CAD build for the part. Positions are in the model's coordinates, mm. Face numbers are marked on the shaded views. A direction names the side the tool comes from. Round coordinates to 2 decimals unless told otherwise and drop trailing zeros. Loops run counter-clockwise (first coordinate to the right, second up) from the corner with the lowest first, then second, coordinate; pieces in that order, holes last. Notation, with made-up numbers: (38.25, -19.5) - (81.25, -19.5) arc R8 cw to (81.25, -10.5) - close; hole circle Ø5 at (-24, 64). An arc over 180 degrees is marked (long way). Use one line per item in the form item = value.
from build123d import *

# Parameters (mm, degrees)
F0_W     = 5.15
F0_H     = 7
F1_DEPTH = 6.74
F2_R     = 1.3
F3_DEPTH = 25
F4_R     = 0.8
F5_DEPTH = 6.741


with BuildPart() as f1:
    # F0 (on Front) → F1 (new body)
    with BuildSketch(Plane.XZ):
        with BuildLine():
            Line((7, 2.5), (-7, 2.5))
            ThreePointArc((-7, 2.5), (-8.06066, 2.06066), (-8.5, 1))
            Line((-8.5, 1), (-8.5, -2.5))
            Line((-8.5, -2.5), (-3.35, -2.5))
            Line((-3.35, -2.5), (3.35, -2.5))
            Line((3.35, -2.5), (8.5, -2.5))
            Line((8.5, -2.5), (8.5, 1))
            ThreePointArc((8.5, 1), (8.06066, 2.06066), (7, 2.5))
        make_face()
        with Locations((-5.925, -6)):
            Rectangle(F0_W, F0_H)
        with Locations((5.925, -6)):
            Rectangle(F0_W, F0_H)
    extrude(amount=F1_DEPTH)

    # F2 (on face) → F3 (cut)
    with BuildSketch(Plane.XZ.offset(6.74)):
        with Locations((-2.6, -3.25)):
            Circle(F2_R)
        with Locations((2.6, -3.25)):
            Circle(F2_R)
    extrude(amount=-F3_DEPTH, mode=Mode.SUBTRACT)

    # F4 (on face) → F5 (cut, through all)
    with BuildSketch(Plane.XZ.offset(6.74)):
        with Locations((-5.925, -4.5)):
            Circle(F4_R)
        with Locations((5.925, -4.5)):
            Circle(F4_R)
    extrude(amount=-F5_DEPTH, mode=Mode.SUBTRACT)


solid = f1.part
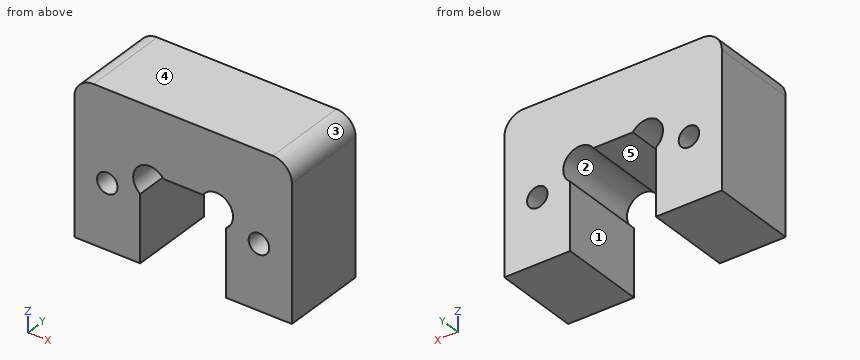
1) Slice it at B-B (z = -7.5). Write the cut outline in (x, y), plus the area to 3 significant figures.
Report:
outline = (-8.5, -6.74) - (-3.35, -6.74) - (-3.35, 0) - (-8.5, 0) - close; (3.35, -6.74) - (8.5, -6.74) - (8.5, 0) - (3.35, 0) - close
area = 69.4 mm^2
2) Tool access for the marked faces 1 and 2: list every direction of +Z, -Z, +X, -X, +Y, -Y with a clear straight run to the whole face (end or side of a thin tool).
Report:
face_1 = -Z, +Y, -Y
face_2 = +Y, -Y
3) Slice it at D-D (x = 6.5). Write the cut outline in (y, z), plus the area to 3 significant figures.
Report:
outline = (-6.74, -9.5) - (0, -9.5) - (0, -5.06) - (-6.74, -5.06) - close; (-6.74, -3.94) - (0, -3.94) - (0, 2.5) - (-6.74, 2.5) - close
area = 73.4 mm^2
4) Two-plate mould, pull along X, no slides. Class the marked faces 3, 4 and 5: +X half, -X half, draft (parallel to the pull), parting line (faces both ways), or undercut.
Report:
face_3 = +X half
face_4 = draft
face_5 = undercut
5) Drill centre lines: probe 1 along X at (y, z) = (-2.5, -9); probe 2 along X at (y, z) = (-3.25, -2.25); probe 3 along Z at (x, y) = (-6, -6). Where is each one in solid material? Low to high.
Report:
probe_1 = -8.5 to -3.35, 3.35 to 8.5
probe_2 = -8.5 to -3.43, -1.77 to 1.77, 3.43 to 8.5
probe_3 = -9.5 to -5.3, -3.7 to 2.5
6) Slice it at A-A (z = -4.5). Write the cut outline in (x, y) (3 decimals).
Report:
outline = (-8.5, -6.74) - (-6.725, -6.74) - (-6.725, 0) - (-8.5, 0) - close; (-5.125, -6.74) - (-3.35, -6.74) - (-3.35, 0) - (-5.125, 0) - close; (3.35, -6.74) - (5.125, -6.74) - (5.125, 0) - (3.35, 0) - close; (6.725, -6.74) - (8.5, -6.74) - (8.5, 0) - (6.725, 0) - close
7) Slice it at C-C (y = -2). Write the cut outline in (x, z) (3 decimals).
Report:
outline = (-8.5, -9.5) - (-3.35, -9.5) - (-3.35, -4.312) arc R1.3 cw (long way) to (-1.538, -2.5) - (1.538, -2.5) arc R1.3 cw (long way) to (3.35, -4.312) - (3.35, -9.5) - (8.5, -9.5) - (8.5, 1) arc R1.5 ccw to (7, 2.5) - (-7, 2.5) arc R1.5 ccw to (-8.5, 1) - close; hole circle Ø1.6 at (-5.925, -4.5); hole circle Ø1.6 at (5.925, -4.5)
8) Flat gauge pin, fed straight in: pin 1 (2.5 mm diameter, centred on x = -0.5, y = -4, fed in from -Z). Where does the tip first touch, or does it go through?
Report:
pin_1 = -2.5
